```python
from build123d import *

# Parameters (mm, degrees)
F0_R     = 11
F1_DEPTH = 3


with BuildPart() as f1:
    # F0 (on Top) → F1 (new body)
    with BuildSketch(Plane.XY):
        with BuildLine():
            ThreePointArc((39.940735, 0), (48.218565, 27.839001), (19.970367, 34.589691))
            ThreePointArc((19.970367, 34.589691), (0, 55.678003), (-19.970367, 34.589691))
            ThreePointArc((-19.970367, 34.589691), (-48.218565, 27.839001), (-39.940735, 0))
            ThreePointArc((-39.940735, 0), (-48.218565, -27.839001), (-19.970367, -34.589691))
            ThreePointArc((-19.970367, -34.589691), (0, -55.678003), (19.970367, -34.589691))
            ThreePointArc((19.970367, -34.589691), (48.218565, -27.839001), (39.940735, 0))
        make_face()
        with Locations((0, -40)):
            Circle(F0_R, mode=Mode.SUBTRACT)
        with Locations((-34.641016, -20)):
            Circle(F0_R, mode=Mode.SUBTRACT)
        with BuildLine():
            ThreePointArc((-5.759242, -16.525167), (-8.429472, -17.541189), (-10.927689, -18.927313))
            ThreePointArc((-10.927689, -18.927313), (-10.97638, -16.070731), (-11.431593, -13.250233))
            ThreePointArc((-11.431593, -13.250233), (-10.135662, -14.265986), (-8.75, -15.155445))
            ThreePointArc((-8.75, -15.155445), (-7.286876, -15.910734), (-5.759242, -16.525167))
        make_face(mode=Mode.SUBTRACT)
        with BuildLine():
            ThreePointArc((11.431593, -13.250233), (10.97638, -16.070731), (10.927689, -18.927313))
            ThreePointArc((10.927689, -18.927313), (8.429472, -17.541189), (5.759242, -16.525167))
            ThreePointArc((5.759242, -16.525167), (7.286876, -15.910734), (8.75, -15.155445))
            ThreePointArc((8.75, -15.155445), (10.135662, -14.265986), (11.431593, -13.250233))
        make_face(mode=Mode.SUBTRACT)
        with BuildLine():
            ThreePointArc((17.190835, 3.274934), (19.405852, 1.470458), (21.855379, 0))
            ThreePointArc((21.855379, 0), (19.405852, -1.470458), (17.190835, -3.274934))
            ThreePointArc((17.190835, -3.274934), (17.422537, -1.644747), (17.5, 0))
            ThreePointArc((17.5, 0), (17.422537, 1.644747), (17.190835, 3.274934))
        make_face(mode=Mode.SUBTRACT)
        with Locations((34.641016, -20)):
            Circle(F0_R, mode=Mode.SUBTRACT)
        with Locations((-34.641016, 20)):
            Circle(F0_R, mode=Mode.SUBTRACT)
        with BuildLine():
            ThreePointArc((-17.190835, -3.274934), (-19.405852, -1.470458), (-21.855379, 0))
            ThreePointArc((-21.855379, 0), (-19.405852, 1.470458), (-17.190835, 3.274934))
            ThreePointArc((-17.190835, 3.274934), (-17.422537, 1.644747), (-17.5, 0))
            ThreePointArc((-17.5, 0), (-17.422537, -1.644747), (-17.190835, -3.274934))
        make_face(mode=Mode.SUBTRACT)
        with BuildLine():
            ThreePointArc((-5.5, 9.526279), (0, 11), (5.5, 9.526279))
            ThreePointArc((5.5, 9.526279), (9.526279, 5.5), (11, 0))
            ThreePointArc((11, 0), (9.526279, -5.5), (5.5, -9.526279))
            ThreePointArc((5.5, -9.526279), (0, -11), (-5.5, -9.526279))
            ThreePointArc((-5.5, -9.526279), (-9.526279, -5.5), (-11, 0))
            ThreePointArc((-11, 0), (-9.526279, 5.5), (-5.5, 9.526279))
        make_face(mode=Mode.SUBTRACT)
        with BuildLine():
            ThreePointArc((-10.927689, 18.927313), (-8.429472, 17.541189), (-5.759242, 16.525167))
            ThreePointArc((-5.759242, 16.525167), (-7.286876, 15.910734), (-8.75, 15.155445))
            ThreePointArc((-8.75, 15.155445), (-10.135662, 14.265986), (-11.431593, 13.250233))
            ThreePointArc((-11.431593, 13.250233), (-10.97638, 16.070731), (-10.927689, 18.927313))
        make_face(mode=Mode.SUBTRACT)
        with Locations((0, 40)):
            Circle(F0_R, mode=Mode.SUBTRACT)
        with BuildLine():
            ThreePointArc((8.75, 15.155445), (7.286876, 15.910734), (5.759242, 16.525167))
            ThreePointArc((5.759242, 16.525167), (8.429472, 17.541189), (10.927689, 18.927313))
            ThreePointArc((10.927689, 18.927313), (10.97638, 16.070731), (11.431593, 13.250233))
            ThreePointArc((11.431593, 13.250233), (10.135662, 14.265986), (8.75, 15.155445))
        make_face(mode=Mode.SUBTRACT)
        with Locations((34.641016, 20)):
            Circle(F0_R, mode=Mode.SUBTRACT)
    extrude(amount=F1_DEPTH)


solid = f1.part
```
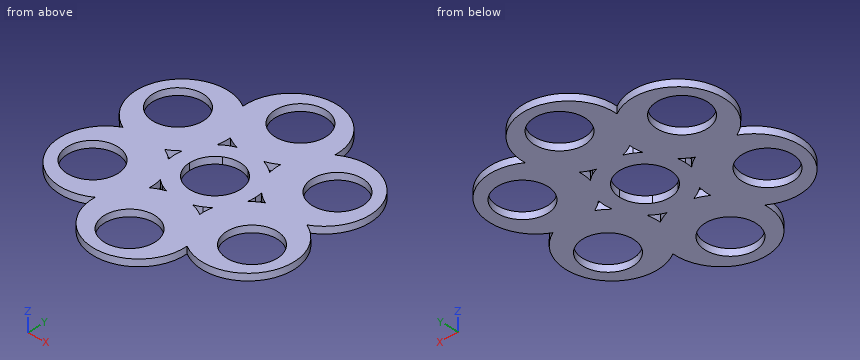
For this review, take the finished solid that the model builds, in its own axes (mm). Coordinates: 2 decimals unless noted, no trailing zeros. Loops run counter-clockwise (first coordinate to the right, second up) from the corner with the lowest first, then second, coordinate; pieces in that order, holes last. Notation, with made-up numbers: (2.5, 75) - (32.5, 75) arc R12 cw to (32.5, 79) - close; hole circle Ø7 at (-40, -28). An arc over 180 degrees is marked (long way). Use one line per item in the form item = value. Start each with the question number.
1) Take a section at D-D (y = -24.5). State the section outline as (x, z) points.
2) Take a section at C-C (x = -30). State the section outline as (y, z) points, plus the area to 3 significant figures.
3) Take a section at A-A (x = 0). State the section outline as (y, z) points.
4) To check wall thickness, follow probe 1 along Y at (x, z) = (0, 1.95); probe 2 along Y at (x, z) = (-39, 2.75); probe 3 along Y at (x, z) = (-25.5, 0.95). State the ranges of each line that lie inside material, in increasing order. Write a range as from..to.
5) Take a section at B-B (y = 40). State the section outline as (x, z) points.
6) For pin 1 (1.5 mm diameter, centred on y = -19.5, z = 1.5, fed in from -X), flat-tipped, find the tip position at first contact; note if it passes through.
From the geometry:
q1.outline = (-49.76, 0) - (-44.68, 0) - (-44.68, 3) - (-49.76, 3) - close; (-24.6, 0) - (24.6, 0) - (24.6, 3) - (-24.6, 3) - close; (44.68, 0) - (49.76, 0) - (49.76, 3) - (44.68, 3) - close
q2.outline = (-37.82, 0) - (-29.97, 0) - (-29.97, 3) - (-37.82, 3) - close; (-10.03, 0) - (10.03, 0) - (10.03, 3) - (-10.03, 3) - close; (29.97, 0) - (37.82, 0) - (37.82, 3) - (29.97, 3) - close
q2.area = 107 mm2
q3.outline = (-55.68, 0) - (-51, 0) - (-51, 3) - (-55.68, 3) - close; (-29, 0) - (-11, 0) - (-11, 3) - (-29, 3) - close; (11, 0) - (29, 0) - (29, 3) - (11, 3) - close; (51, 0) - (55.68, 0) - (55.68, 3) - (51, 3) - close
q4.probe_1 = -55.68..-51, -29..-11, 11..29, 51..55.68
q4.probe_2 = -36.12..-30.1, -9.9..9.9, 30.1..36.12
q4.probe_3 = -37.1..-26.12, -13.88..13.88, 26.12..37.1
q5.outline = (-19.53, 0) - (-11, 0) - (-11, 3) - (-19.53, 3) - close; (11, 0) - (19.53, 0) - (19.53, 3) - (11, 3) - close
q6.pin_1 = -50.88
